Here's how the part is built. I have some questions about the finished solid (model axes, mm). A direction names the side the tool comes from. Give positions to 0.01 mm unless a question says otherwise; leave off trailing zeros. Write each loop counter-clockwise with the first axis right and the second up, starting at its lowest first coordinate (ties: lowest second). Pieces come first, ordered by that corner, then holes. Notation, with made-up numbers: (17.5, 26.25) - (56.5, 26.25) arc R13 cw to (56.5, 39.25) - close; hole circle Ø1 at (8, 45). An arc over 180 degrees is marked (long way). Use a Markdown table: item, result.
```python
from build123d import *

# Parameters (mm, degrees)
SKETCH1_R           = 0.75
BOSS_EXTRUDE1_DEPTH = 5


with BuildPart() as part:
    # Sketch1 → Boss-Extrude1 (new body)
    # profile 1 of 5: a face of its own
    with BuildSketch(Plane.XY):
        with BuildLine():
            Line((-7, -2), (-2, -2))
            Line((-2, -2), (-2, 0))
            Line((-2, 0), (-2, 2))
            Line((-2, 2), (-7, 2))
            ThreePointArc((-7, 2), (-7.280109889, 0), (-7, -2))
        make_face()
    # profile 2 of 5: a face of its own
    with BuildSketch(Plane.XY):
        with BuildLine():
            Line((0, 2), (2, 2))
            Line((2, 2), (2, 7))
            ThreePointArc((2, 7), (0, 7.280109889), (-2, 7))
            Line((-2, 7), (-2, 2))
            Line((-2, 2), (0, 2))
        make_face()
    # profile 3 of 5: a face of its own
    with BuildSketch(Plane.XY):
        Polygon((-2, -2), (0, -2), (2, -2), (2, 0), (2, 2), (0, 2), (-2, 2), (-2, 0), align=None)
        Circle(SKETCH1_R, mode=Mode.SUBTRACT)
    # profile 4 of 5: a face of its own
    with BuildSketch(Plane.XY):
        with BuildLine():
            Line((2, -2), (0, -2))
            Line((0, -2), (-2, -2))
            Line((-2, -2), (-2, -7))
            ThreePointArc((-2, -7), (0, -7.280109889), (2, -7))
            Line((2, -7), (2, -2))
        make_face()
    # profile 5 of 5: a face of its own
    with BuildSketch(Plane.XY):
        with BuildLine():
            Line((2, 0), (2, -2))
            Line((2, -2), (7, -2))
            ThreePointArc((7, -2), (7.20974234, -1.009760064), (7.280109889, 0))
            ThreePointArc((7.280109889, 0), (7.20974234, 1.009760064), (7, 2))
            Line((7, 2), (2, 2))
            Line((2, 2), (2, 0))
        make_face()
    extrude(amount=BOSS_EXTRUDE1_DEPTH)


solid = part.part
```
Item 1: For faces 1 (the flat face through (5, 2, 2)), 2 (the flat face through (-2, -4, 2)), 3 (the flat face through (2, -5, 2)), which set-ups out of +Z, -Z, +X, -X, +Y, -Y let a thin tool reach every point of the face, with its end or its side?
Values:
| item | result |
|---|---|
| face 1 | +Z, -Z, +X, +Y |
| face 2 | +Z, -Z, -X, -Y |
| face 3 | +Z, -Z, +X, -Y |
Item 2: I need wall thicknesses on line 1 along Y through (x, z) = (0, 1.75); line 2 along Y through (x, z) = (4.5, 1.45). Which ranges of each line are inside material? Lowest first, please. Write a range as [from, to].
Values:
| item | result |
|---|---|
| line 1 | y = [-7.28, -0.75], [0.75, 7.28] |
| line 2 | y = [-2, 2] |
Item 3: Thinking about a two-plate mould opening in X: for faces 4 (the flat face through (-4, 2, 2)), 5 (the cylindrical face through (-0.75, 0.03, 2.46)), 6 (the cylindrical face through (0.03, 7.28, 2.46)), which applies, +X half, -X half, draft (parallel to the pull), parting line (faces both ways), or undercut?
Values:
| item | result |
|---|---|
| face 4 | draft |
| face 5 | undercut |
| face 6 | parting line |
Item 4: Will these pins go through, and if not, where does the flat tip stop? pin 1 Ø0.9 at (x, y) = (0, 0) entering from +Z; pin 2 Ø1 at (x, z) = (1, 4.5) entering from -Y; pin 3 Ø2 at (x, z) = (-5.5, 2) entering from +Y; pin 4 Ø1 at (y, z) = (-4, 2.5) entering from +X.
Values:
| item | result |
|---|---|
| pin 1 | passes through |
| pin 2 | stops at y = -7.26 |
| pin 3 | stops at y = 2 |
| pin 4 | stops at x = 2 |
Item 5: If we section it at C-C, the plane x = 5.75: Write out the boundary of the cut face in (y, z), plus the area to 3 significant figures.
Values:
| item | result |
|---|---|
| outline | (-2, 0) - (2, 0) - (2, 5) - (-2, 5) - close |
| area | 20.0 mm2 |
Item 6: If we section it at B-B, the plane z = 4.45: Write out the boundary of the cut face in (x, y), plus the area to 3 significant figures.
Values:
| item | result |
|---|---|
| outline | (-7, -2) - (-2, -2) - (-2, -7) arc R7.28 ccw to (2, -7) - (2, -2) - (7, -2) arc R7.28 ccw to (7, 2) - (2, 2) - (2, 7) arc R7.28 ccw to (-2, 7) - (-2, 2) - (-7, 2) arc R7.28 ccw to start; hole circle Ø1.5 at (0, 0) |
| area | 97.2 mm2 |
Item 7: If we section it at A-A, the plane x = 0: Write out the boundary of the cut face in (y, z), plus the area to 3 significant figures.
Values:
| item | result |
|---|---|
| outline | (-7.28, 0) - (-0.75, 0) - (-0.75, 5) - (-7.28, 5) - close; (0.75, 0) - (7.28, 0) - (7.28, 5) - (0.75, 5) - close |
| area | 65.3 mm2 |
